For this review, take the finished solid that the model builds, in its own axes (mm). A direction names the side the tool comes from. Coordinates: 2 decimals unless noted, no trailing zeros. Write each loop counter-clockwise with the first axis right and the second up, starting at its lowest first coordinate (ties: lowest second). Pieces come first, ordered by that corner, then holes.
```python
from build123d import *

# Parameters (mm, degrees)
FILLET1_R = 9.652
FILLET2_R = 6.35


with BuildPart() as part:
    # Sketch1 → Revolve3 (revolve)
    with BuildSketch(Plane.XY, mode=Mode.PRIVATE) as revolve3_sk:
        Polygon((-101.6, 19.05), (101.6, 19.05), (101.6, 14.2875), (203.2, 14.2875), (203.2, 0), (-177.8, 0), (-177.8, 9.525), (-101.6, 9.525), align=None)
    revolve(revolve3_sk.sketch.rotate(Axis((-177.8, 0, 0), (1, 0, 0)), 90), axis=Axis((-177.8, 0, 0), (1, 0, 0)))

    # Fillet1
    # the kernel refuses this fillet: 9.652 mm, written as the material it adds along each edge
    with BuildSketch(Plane(origin=(-101.6, 0, 0), x_dir=(0, 0, 1), z_dir=(0, 1, 0))) as fillet1_piece_1_section:
        with BuildLine():
            CenterArc((9.525 + FILLET1_R, -FILLET1_R), FILLET1_R, 90, 90)
            Line((9.525 + FILLET1_R, 0), (9.525, 0))
            Line((9.525, 0), (9.525, -FILLET1_R))
        make_face()
    fillet1_piece_1 = revolve(axis=Axis((-101.6, 0, 0), (1, 0, 0)), mode=Mode.PRIVATE)
    fillet1_piece_1 = fillet1_piece_1 & Plane(origin=(-104.387487572, 0, 0), x_dir=(0, 0, 1), z_dir=(1, 0, 0)) * Cylinder(19.05, 77, mode=Mode.PRIVATE)
    add(fillet1_piece_1)

    # Fillet2
    # the kernel refuses this fillet: 6.35 mm, written as the material it adds along each edge
    with BuildSketch(Plane(origin=(101.6, 0, 0), x_dir=(0, 0, 1), z_dir=(0, 1, 0))) as fillet2_piece_1:
        with BuildLine():
            CenterArc((20.6375, 6.148361062), FILLET2_R, 180, 75.522487814)
            Line((14.2875, 6.148361062), (14.1605, 6.148361062))
            Line((14.1605, 6.148361062), (14.1605, 0))
            Line((14.1605, 0), (14.2875, -0.127))
            ThreePointArc((14.2875, -0.127), (16.66875, -0.127), (19.01825, -0.122967221))
            Line((19.01825, -0.122967221), (19.05, 0))
        make_face()
    revolve(axis=Axis((101.6, 0, 0), (1, 0, 0)))


solid = part.part
```
Q1. Tool access review of faces 1 (the cylindrical face through (1.42, 11.59, -15.12)), 2 (the cylindrical face through (-144.06, 9.3, -2.06)), 3 (the cylindrical face through (156.142, -0.628, -14.274)): name each direction out of +Z, -Z, +X, -X, +Y, -Y from which nothing blocks a thin tool from reaching the whole face with its end or side.
Ans:
face 1: +X, -X
face 2: -X
face 3: +X
Q2. For probe 1 along Z at (x, y) = (177.5, 1); probe 2 along Z at (x, y) = (94, 0.5), list the stretches that pass through material, from the lowest coordinate up.
Ans:
probe 1: z = -14.25 to 14.25
probe 2: z = -19.04 to 19.04
Q3. Clearance check with flat-ended pins moving along their axes: pin 1 Ø3 at (x, z) = (-93, 10) entering from -Y; pin 2 Ø2 at (x, y) = (154, 14) entering from -Z; pin 3 Ø4 at (x, z) = (44.5, 14.5) entering from +Y. State where each tip first meets the part, or that it passes through.
Ans:
pin 1: stops at y = -17.05
pin 2: stops at z = -5.93
pin 3: stops at y = 14.38
Q4. Add section D-D (x = 175.5). State the section outline as (y, z) points (1 decimal).
Ans:
outline: circle Ø28.6 at (0, 0)
Q5. Add section C-C (x = -79.5). State the section outline as (y, z) points, then the cut area to 3 significant figures.
Ans:
outline: circle Ø38.1 at (0, 0)
area: 1,140 mm2
